```python
from build123d import *

# Parameters (mm, degrees)
CROQUIS1_R              = 3
SALIENTE_EXTRUIR1_DEPTH = 5
CROQUIS2_OUTSIDE_W      = 22.536
CROQUIS2_OUTSIDE_H      = 20.988
CROQUIS2_OUTSIDE_R      = 5
CORTAR_EXTRUIR1_DEPTH   = 5
CORTAR_EXTRUIR1_DRAFT   = -30
CROQUIS3_OUTSIDE_W      = 22.536
CROQUIS3_OUTSIDE_H      = 20.988
CROQUIS3_OUTSIDE_R      = 5
CORTAR_EXTRUIR2_DEPTH   = 5
CORTAR_EXTRUIR2_DRAFT   = -30


with BuildPart() as part:
    # Croquis1 → Saliente-Extruir1 (new body)
    with BuildSketch(Plane.XY):
        Polygon((5.773502692, 0), (2.886751346, 5), (-2.886751346, 5), (-5.773502692, 0), (-2.886751346, -5), (2.886751346, -5), align=None)
        Circle(CROQUIS1_R, mode=Mode.SUBTRACT)
    extrude(amount=SALIENTE_EXTRUIR1_DEPTH)


with BuildPart() as cortar_extruir1_tool:
    # Croquis2 outside → Cortar-Extruir1 (with draft: the straight prism first)
    with BuildSketch(Plane.XY.offset(5)):
        Rectangle(CROQUIS2_OUTSIDE_W, CROQUIS2_OUTSIDE_H)
        Circle(CROQUIS2_OUTSIDE_R, mode=Mode.SUBTRACT)
    extrude(amount=-CORTAR_EXTRUIR1_DEPTH)
    # Cortar-Extruir1: the draft: its side faces are tilted about the plane it starts from
    cortar_extruir1_sides = [cortar_extruir1_tool.faces().sort_by_distance(p)[0] for p in [
        (0, -10.494, 2.5),
        (11.268, 0, 2.5),
        (0, 10.494, 2.5),
        (-11.268, 0, 2.5),
        (-5, 0, 2.5),
    ]]
    draft(cortar_extruir1_sides, Plane.XY.offset(5), CORTAR_EXTRUIR1_DRAFT)


with BuildPart() as part_1:
    add(part.part)

    # Cortar-Extruir1: cut by cortar_extruir1_tool
    add(cortar_extruir1_tool.part, mode=Mode.SUBTRACT)


with BuildPart() as cortar_extruir2_tool:
    # Croquis3 outside → Cortar-Extruir2 (with draft: the straight prism first)
    with BuildSketch(Plane(origin=(0, 0, 0), x_dir=(-1, 0, 0), z_dir=(0, 0, -1))):
        Rectangle(CROQUIS3_OUTSIDE_W, CROQUIS3_OUTSIDE_H)
        Circle(CROQUIS3_OUTSIDE_R, mode=Mode.SUBTRACT)
    extrude(amount=-CORTAR_EXTRUIR2_DEPTH)
    # Cortar-Extruir2: the draft: its side faces are tilted about the plane it starts from
    cortar_extruir2_sides = [cortar_extruir2_tool.faces().sort_by_distance(p)[0] for p in [
        (0, -10.494, 2.5),
        (-11.268, 0, 2.5),
        (0, 10.494, 2.5),
        (11.268, 0, 2.5),
        (5, 0, 2.5),
    ]]
    draft(cortar_extruir2_sides, Plane(origin=(0, 0, 0), x_dir=(-1, 0, 0), z_dir=(0, 0, -1)), CORTAR_EXTRUIR2_DRAFT)


with BuildPart() as part_2:
    add(part_1.part)

    # Cortar-Extruir2: cut by cortar_extruir2_tool
    add(cortar_extruir2_tool.part, mode=Mode.SUBTRACT)


solid = part_2.part
```
The model under review builds one solid part; all positions refer to its coordinate system, in mm. Coordinates: 2 decimals unless noted, no trailing zeros. Order: outer loops, then holes, each group sorted by start corner. A loop starts at its lowest first (then second) coordinate and runs counter-clockwise, first axis right, second up. Notation, with made-up numbers: M 27,68.5 L 38,68.5 A15 ccw 38,76.5 Z; hole C 44,77 d5. An arc over 180 degrees is marked long. One line per question, with ' | ' between items.
(1) Add section A-A, the plane z = 1.55. Write out the cut boundary in (x, y).
Geometry results:
outline: M -5.77,0 L -2.89,-5 L 2.89,-5 L 5.77,0 L 2.89,5 L -2.89,5 Z; hole C 0,0 d6
(2) For probe 1 along Y at (x, z) = (0, 2.35); probe 2 along Y at (x, z) = (-1.75, 3.15); probe 3 along X at (y, z) = (-1.75, 3.5), list the stretches that pass through material, from the lowest coordinate up. Write a range as from..to.
Geometry results:
probe 1: y = -5..-3, 3..5 | probe 2: y = -5..-2.44, 2.44..5 | probe 3: x = -4.76..-2.44, 2.44..4.76
(3) The part is to be moulded in two halves that separate along X. For faces 1 (the face through (3.3, 0.1, 0)), 2 (the face through (-2.581, 4.496, 4.681)), 3 (the face through (-3, 0, 2)), say which applies: +X half, -X half, draft (parallel to the pull), parting line (faces both ways), or undercut.
Geometry results:
face 1: draft | face 2: -X half | face 3: undercut
(4) Add section B-B, the plane z = 0.6. Write out the cut boundary in (x, y), then the cut area to 3 significant figures.
Geometry results:
outline: M -5.28,-0.86 L -3.38,-4.14 A5.35 ccw -1.89,-5 L 1.89,-5 A5.35 ccw 3.38,-4.14 L 5.28,-0.86 A5.35 ccw 5.28,0.86 L 3.38,4.14 A5.35 ccw 1.89,5 L -1.89,5 A5.35 ccw -3.38,4.14 L -5.28,0.86 A5.35 ccw Z; hole C 0,0 d6 | area: 56.2 mm²
(5) Insertion check: pin 1 (3 mm diameter, centred on y = 0, z = 1, fed in from -X); pin 2 (2 mm diameter, centred on y = -2.5, z = 1.5, fed in from +X). Each pin has a flat end and moves straight along its axis. Give the tip position at first contact, or say it passes through.
Geometry results:
pin 1: stops at x = -5.77 | pin 2: stops at x = 4.91
